Could you check a few things on this drawing? It's one solid part, dimensions in mm from its lowest x, y, z. A direction names the side the tool comes from. Give positions to 0.01 mm unless a question says otherwise; leave off trailing zeros. Order: outer loops, then holes, each group sorted by start corner. A loop starts at its lowest first (then second) coordinate and runs counter-clockwise, first axis right, second up.
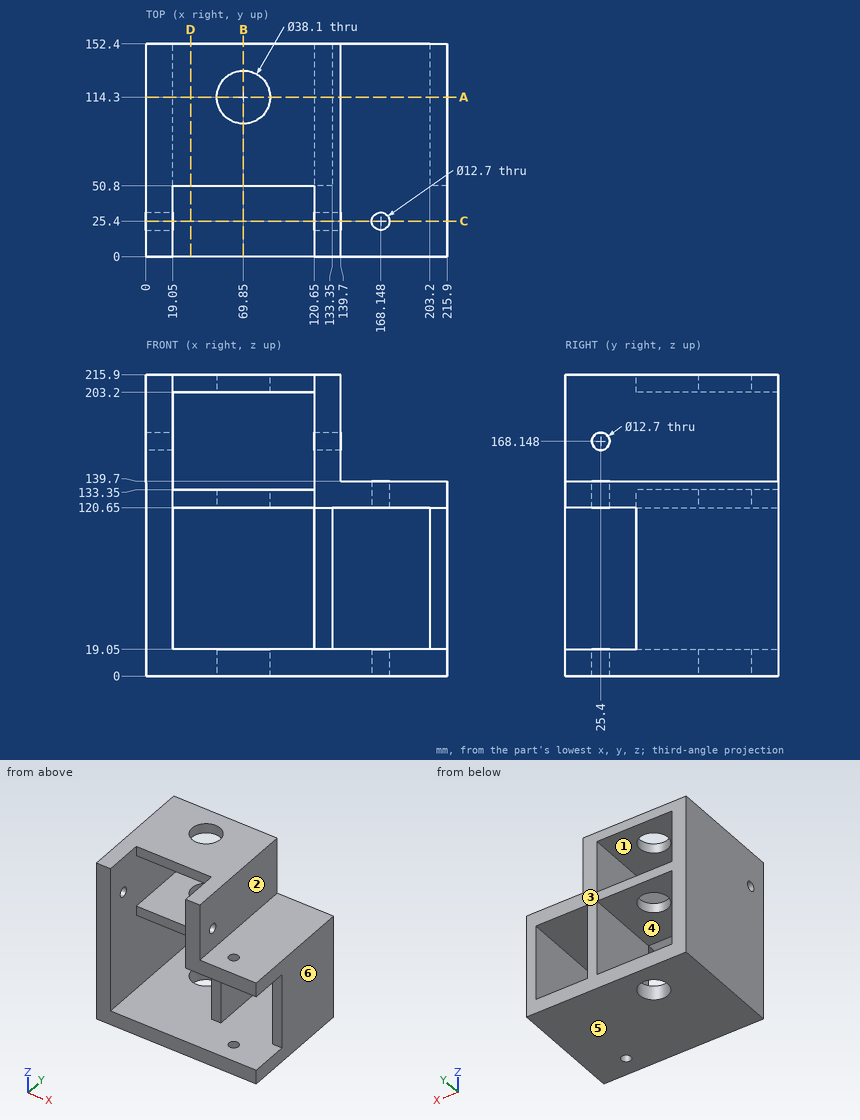
1) Suppose I cut it at C-C (y = 25.4). Please give me the cut outline in (x, z), and give its area (3 significant figures).
2) Which directions (+Z, -Z, +X, -X, +Y, -Y) give clear straight access to the entire face, cutting with the end or side of a thin tool? Please do the marked faces 1, 2 and 3.
3) Suppose I cut it at B-B (x = 69.85). Please give me the cut outline in (y, z).
4) Suppose I cut it at D-D (x = 32). Please give me the cut outline in (y, z), and give its area (3 significant figures).
5) If I drill on line 1 (Z direction, x = 108, y = 60.5); line 2 (Z direction, x = 189.5, y = 19), over which ranges is the centre line in solid material (lowest first)?
6) I'm going to push flat-ended pins straight in: pin 1 Ø6 at (y, z) = (95, 152.5) entering from +X; pin 2 Ø4 at (x, z) = (49.5, 208.5) entering from -Y; pin 3 Ø3 at (x, y) = (192.5, 69.5) entering from +Z. Where does each tip first touch, or does it pass through?
7) Suppose I cut it at A-A (y = 114.3). Give the number of separate pieces and of enclosed holes in the cut face, and give its area (3 significant figures).
8) We'd pull the mould along X, two halves only. Please class the marked faces 4, 5 and 6: +X half, -X half, draft (parallel to the pull), parting line (faces both ways), or undercut.
Results:
1. outline: (0, 0) - (161.8, 0) - (161.8, 19.05) - (19.05, 19.05) - (19.05, 161.8) - (0, 161.8) - close; (0, 174.5) - (19.05, 174.5) - (19.05, 215.9) - (0, 215.9) - close; (120.65, 120.65) - (161.8, 120.65) - (161.8, 139.7) - (139.7, 139.7) - (139.7, 161.8) - (120.65, 161.8) - close; (120.65, 174.5) - (139.7, 174.5) - (139.7, 215.9) - (120.65, 215.9) - close; (174.5, 0) - (215.9, 0) - (215.9, 19.05) - (174.5, 19.05) - close; (174.5, 120.65) - (215.9, 120.65) - (215.9, 139.7) - (174.5, 139.7) - close
1. area: 10,200 mm2
2. face 1: +Y, -Y
2. face 2: +Z, +X, +Y, -Y
2. face 3: +Z, -Z, +X, -X, +Y
3. outline: (0, 0) - (95.25, 0) - (95.25, 19.05) - (0, 19.05) - close; (50.8, 120.65) - (95.25, 120.65) - (95.25, 133.35) - (50.8, 133.35) - close; (50.8, 203.2) - (95.25, 203.2) - (95.25, 215.9) - (50.8, 215.9) - close; (133.35, 0) - (152.4, 0) - (152.4, 19.05) - (133.35, 19.05) - close; (133.35, 120.65) - (152.4, 120.65) - (152.4, 133.35) - (133.35, 133.35) - close; (133.35, 203.2) - (152.4, 203.2) - (152.4, 215.9) - (133.35, 215.9) - close
4. outline: (0, 0) - (152.4, 0) - (152.4, 19.05) - (0, 19.05) - close; (50.8, 120.65) - (152.4, 120.65) - (152.4, 133.35) - (50.8, 133.35) - close; (50.8, 203.2) - (152.4, 203.2) - (152.4, 215.9) - (50.8, 215.9) - close
4. area: 5,480 mm2
5. line 1: z = 0 to 19.05, 120.65 to 133.35, 203.2 to 215.9
5. line 2: z = 0 to 19.05, 120.65 to 139.7
6. pin 1: stops at x = 139.7
6. pin 2: stops at y = 50.8
6. pin 3: stops at z = 139.7
7. separate pieces: 2
7. enclosed holes: 1
7. area: 14,600 mm2
8. face 4: undercut
8. face 5: draft
8. face 6: +X half
